from build123d import *

# Parameters (mm, degrees)
ESQUISSE1_W        = 57
ESQUISSE1_H        = 57
ESQUISSE1_R        = 2.5
BOSS_EXTRU_1_DEPTH = 4.5
CONG_2_R           = 5
ESQUISSE2_R        = 19
BOSS_EXTRU_2_DEPTH = 1
CHANFREIN1_SIZE    = 1
ESQUISSE3_R        = 28.5
BOSS_EXTRU_3_DEPTH = 48
ESQUISSE4_R        = 6.75
BOSS_EXTRU_4_DEPTH = 1.5
ESQUISSE5_R        = 3
BOSS_EXTRU_5_DEPTH = 20


with BuildPart() as part:
    # Esquisse1 → Boss.-Extru.1 (new body)
    with BuildSketch(Plane.XY):
        with Locations((-1.798558634, -6.791590494)):
            Rectangle(ESQUISSE1_W, ESQUISSE1_H)
        with Locations((-25.798558634, 17.208409506)):
            Circle(ESQUISSE1_R, mode=Mode.SUBTRACT)
        with Locations((22.201441366, 17.208409506)):
            Circle(ESQUISSE1_R, mode=Mode.SUBTRACT)
        with Locations((22.201441366, -30.791590494)):
            Circle(ESQUISSE1_R, mode=Mode.SUBTRACT)
        with Locations((-25.798558634, -30.791590494)):
            Circle(ESQUISSE1_R, mode=Mode.SUBTRACT)
    extrude(amount=BOSS_EXTRU_1_DEPTH)

    # Congé2
    cong_2_edges = [part.edges().sort_by_distance(p)[0] for p in [
        (-30.298558634, 21.708409506, 2.25),
        (26.701441366, 21.708409506, 2.25),
        (26.701441366, -35.291590494, 2.25),
        (-30.298558634, -35.291590494, 2.25),
    ]]
    fillet(cong_2_edges, radius=CONG_2_R)

    # Esquisse2 → Boss.-Extru.2 (add)
    with BuildSketch(Plane(origin=(0, 0, 0), x_dir=(-1, 0, 0), z_dir=(0, 0, -1))):
        with Locations(Location((1.798558634, -6.791590494, 0), (0, 0, 180))):
            Circle(ESQUISSE2_R)
    extrude(amount=BOSS_EXTRU_2_DEPTH)

    # Chanfrein1
    chanfrein1_edges = [part.edges().sort_by_distance(p)[0] for p in [
        (-20.798558634, -6.791590494, -1),
    ]]
    chamfer(chanfrein1_edges, length=CHANFREIN1_SIZE - 0.0001)  # a hair under: the kernel refuses the full size

    # Esquisse3 → Boss.-Extru.3 (add)
    with BuildSketch(Plane.XY.offset(4.5)):
        with Locations((-1.798558634, -6.791590494)):
            Circle(ESQUISSE3_R)
    extrude(amount=BOSS_EXTRU_3_DEPTH)

    # Esquisse4 → Boss.-Extru.4 (add)
    with BuildSketch(Plane(origin=(0, 0, -1), x_dir=(-1, 0, 0), z_dir=(0, 0, -1))):
        with Locations((1.798558634, -6.791590494)):
            Circle(ESQUISSE4_R)
    extrude(amount=BOSS_EXTRU_4_DEPTH)

    # Esquisse5 → Boss.-Extru.5 (add)
    with BuildSketch(Plane(origin=(0, 0, -2.5), x_dir=(-1, 0, 0), z_dir=(0, 0, -1))):
        with Locations((1.798558634, -6.791590494)):
            Circle(ESQUISSE5_R)
    extrude(amount=BOSS_EXTRU_5_DEPTH)


solid = part.part
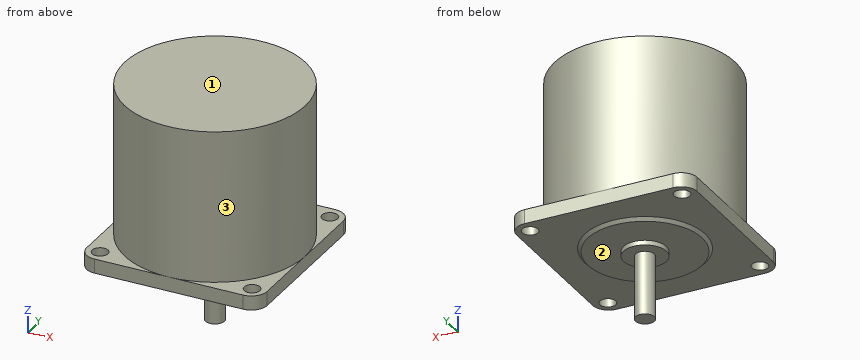
Work out the finished part from the listing and answer in its coordinate system (mm). Face numbers are marked on the shaded views. A direction names the side the tool comes from. Round coordinates to 2 decimals unless told otherwise and drop trailing zeros. Loops run counter-clockwise (first coordinate to the right, second up) from the corner with the lowest first, then second, coordinate; pieces in that order, holes last. Notation, with made-up numbers: (29.5, 9) -> (81.5, 9) arc R20 ccw to (81.5, 37) -> close; hole circle Ø10 at (-3.75, -3.5). An arc over 180 degrees is marked (long way). Use one line per item in the form item = value.
(1) Straight lines are drawn through the part: line 1 (Z direction, x = 18.5, y = -17); line 2 (Z direction, x = -18, y = -11.5); line 3 (X direction, y = 14, z = 38). For each, find the intervals that lie inside material, in ascending order.
Answer list:
line_1 = 0 to 52.5
line_2 = -1 to 52.5
line_3 = -21.29 to 17.69
(2) A tool of negligible diameter and unlimited length cuts with its end or side. For the marked faces 1, 2 and 3, from which of +Z, -Z, +X, -X, +Y, -Y can it reach the whole face along a straight path? Write none if from no direction.
Answer list:
face_1 = +Z, +X, -X, +Y, -Y
face_2 = -Z
face_3 = +Z
(3) Find section A-A on z = -7. Give the vertices of the cut face in (x, y).
Answer list:
outline = circle Ø6 at (-1.8, -6.79)
(4) Flat-ended cylindrical pins translate along their axes: P1, Ø2, axis at x = 6.5, z = 10.5, coming from the -Y side; P2, Ø10, axis at x = -20, z = 37.5, coming from the +Y side; P3, Ø3, axis at x = 19.5, y = 14.5, coming from the -Z side; P4, Ø3, axis at x = 22.2, y = -30.79, coming from the -Z side. Find the tip coordinate at first contact, or state that the pin passes through.
Answer list:
P1 = -34.34
P2 = 18.47
P3 = 0
P4 = through
(5) Find section B-B on z = 25. Give the vertices of the cut face in (x, y).
Answer list:
outline = circle Ø57 at (-1.8, -6.79)
